Read the model definition and answer for the solid it produces. Units are mm, in the model's axes. A direction names the side the tool comes from. Coordinates: 2 decimals unless noted, no trailing zeros. Write each loop counter-clockwise with the first axis right and the second up, starting at its lowest first coordinate (ties: lowest second). Pieces come first, ordered by that corner, then holes.
(1) Which of the six approach directions +Z, -Z, +X, -X, +Y, -Y give full straight-line access (tool end or side, diameter ignored) to faces 1 (the flat face through (1.8, 1, 11)), 2 (the flat face through (-11, 1, -1.8)), 3 (the flat face through (-8, 2.5, 8)), 4 (the flat face through (9, 2.5, -9))?
(2) Given pin 1 (6 mm diameter, centred on y = -2, z = 5, fed in from -X); pin 2 (6 mm diameter, centred on x = -1.5, z = 2, fed in from +Y); pin 3 (0.6 mm diameter, centred on x = 0.5, z = 11, fed in from -Y); pin 4 (3 mm diameter, centred on x = -8.5, z = 7.5, fed in from +Y), each flat-ended and moving along its own axis, determine where each tip first touches the part or whether it passes through.
(3) Section A-A on y = -1.25 is taken. Write down the section's boundary in (x, z), then the cut area to 3 significant figures.
(4) Find the intervals of material crossed by probe 1 along Y at (x, z) = (7.25, 3); probe 2 along Y at (x, z) = (1.5, -3); probe 3 along X at (y, z) = (-0.75, 8.25), in increasing order.
from build123d import *

# Parameters (mm, degrees)
PAD011_DEPTH    = 2.8
SKETCH021_W     = 23.1
SKETCH021_H     = 23.1
PAD012_DEPTH    = 5
SKETCH023_R     = 2.5
PAD013_DEPTH    = 3
FILLET_R        = 2
FILLET001_R     = 7
SKETCH025_R     = 10.55
PAD014_DEPTH    = 9
PAD014_TAPER    = 2
CHAMFER006_SIZE = 1


with BuildPart() as part:
    # Sketch020 → Pad011 (new body)
    with BuildSketch(Plane.XZ):
        Polygon((-1.8, 11.55), (-1.8, 1.8), (-11.55, 1.8), (-11.55, -1.8), (-1.8, -1.8), (-1.8, -11.55), (1.8, -11.55), (1.8, -1.8), (11.55, -1.8), (11.55, 1.8), (1.8, 1.8), (1.8, 11.55), align=None)
    extrude(amount=PAD011_DEPTH)

    # Sketch021 → Pad012 (join)
    with BuildSketch(Plane.XZ):
        Rectangle(SKETCH021_W, SKETCH021_H)
    extrude(amount=-PAD012_DEPTH)

    # Sketch023 (on Face7 of Pad012) → Pad013 (join)
    with BuildSketch(Plane(origin=(0, 5, 0), x_dir=(1, 0, 0), z_dir=(0, 1, 0))):
        Circle(SKETCH023_R)
    extrude(amount=PAD013_DEPTH)

    # Fillet
    fillet_edges = [part.edges().sort_by_distance(p)[0] for p in [
        (-2.5, 8, 0),
    ]]
    fillet(fillet_edges, radius=FILLET_R)

    # Fillet001
    fillet001_edges = [part.edges().sort_by_distance(p)[0] for p in [
        (-2.5, 5, 0),
    ]]
    fillet(fillet001_edges, radius=FILLET001_R)

    # Sketch025 → Pad014 (join)
    with BuildSketch(Plane.XZ):
        Circle(SKETCH025_R)
    extrude(amount=PAD014_DEPTH, taper=PAD014_TAPER)

    # Chamfer006
    chamfer006_edges = [part.edges().sort_by_distance(p)[0] for p in [
        (-11.55, 2.5, 11.55),
        (-11.55, 2.5, -11.55),
        (11.55, 2.5, 11.55),
        (11.55, 2.5, -11.55),
    ]]
    chamfer(chamfer006_edges, length=CHAMFER006_SIZE)


with BuildPart() as part_1:
    # Body012 placement: moved
    add(part.part.moved(Location((0, 2.5, 0))))


solid = part_1.part
Response:
1. face 1: +Z, +X, -Y
1. face 2: -Z, -X, -Y
1. face 3: +Z, -X, -Y
1. face 4: -Z, +X, -Y
2. pin 1: stops at x = -10.21
2. pin 2: stops at y = 10.5
2. pin 3: stops at y = -0.3
2. pin 4: stops at y = 7.5
3. outline: circle Ø20.84 at (0, 0)
3. area: 341 mm2
4. probe 1: y = -6.5 to 7.5
4. probe 2: y = -6.5 to 8.66
4. probe 3: x = -6.39 to 6.39
